The listing builds one solid part. Answer for the finished solid, in the listing's coordinates (mm). Face numbers are marked on the shaded views. Round coordinates to 2 decimals unless told otherwise and drop trailing zeros. Write each loop counter-clockwise with the first axis right and the second up, starting at its lowest first coordinate (ties: lowest second). Pieces come first, ordered by that corner, then holes. Notation, with made-up numbers: (-34.5, -18) - (16.5, -18) arc R19 ccw to (16.5, -10) - close; hole circle Ø9 at (84, -20.5). An arc over 180 degrees is marked (long way). Answer in a Markdown table with one row per item.
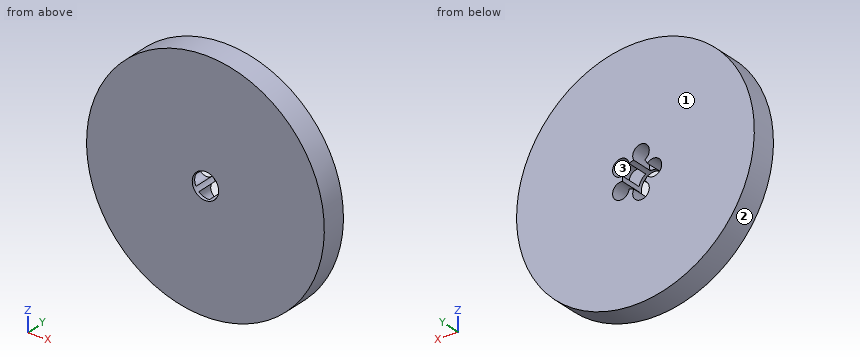
from build123d import *

# Parameters (mm, degrees)
SKETCH1_R           = 90
BOSS_EXTRUDE1_DEPTH = 19
SKETCH2_R           = 10
CUT_EXTRUDE1_DEPTH  = 129.689548915
SKETCH3_R           = 6.277196243
CUT_EXTRUDE2_DEPTH  = 16.549655
CIRPATTERN1_START   = 2.450345027
CIRPATTERN1_DEPTH   = 16.549654973


# Read off the part's stored shape, not the designer's step: CirPattern1
with BuildPart() as part:
    # Sketch1 → Boss-Extrude1 (new body)
    with BuildSketch(Plane(origin=(0, 0, 0), x_dir=(1, 0, 0), z_dir=(0, 1, 0))):
        with Locations(Location((0, 0, 0), (0, 0, 270))):
            Circle(SKETCH1_R)
    extrude(amount=BOSS_EXTRUDE1_DEPTH)

    # Sketch2 → Cut-Extrude1 (cut, through all)
    with BuildSketch(Plane(origin=(0, 0, 0), x_dir=(1, 0, 0), z_dir=(0, 1, 0))):
        with Locations(Location((0, 0, 0), (0, 0, 270))):
            Circle(SKETCH2_R)
    extrude(amount=CUT_EXTRUDE1_DEPTH, mode=Mode.SUBTRACT)

    # Sketch3 → Cut-Extrude2 (cut)
    with BuildSketch(Plane(origin=(0, 19, 0), x_dir=(1, 0, 0), z_dir=(0, 1, 0))):
        with Locations((-13.61267623, 0)):
            Circle(SKETCH3_R)
    extrude(amount=-CUT_EXTRUDE2_DEPTH, mode=Mode.SUBTRACT)

    # CirPattern1 outline → CirPattern1 (cut)
    with BuildSketch(Plane(origin=(0, 0, 0), x_dir=(1, 0, 0), z_dir=(0, 1, 0)).offset(CIRPATTERN1_START)):
        with BuildLine():
            ThreePointArc((1.290880947, -9.916331296), (-3.090169944, -9.510565163), (-6.873017917, -7.263719758))
            ThreePointArc((-6.873017917, -7.263719758), (-6.146308609, -18.916392824), (1.290880947, -9.916331296))
        make_face()
        with BuildLine():
            ThreePointArc((1.290880947, 9.916331296), (-6.146308609, 18.916392824), (-6.873017917, 7.263719758))
            ThreePointArc((-6.873017917, 7.263719758), (-3.090169944, 9.510565163), (1.290880947, 9.916331296))
        make_face()
        with BuildLine():
            ThreePointArc((9.829895648, -1.836614156), (8.090169944, -5.877852523), (4.784328669, -8.781241324))
            ThreePointArc((4.784328669, -8.781241324), (16.091244847, -11.69097371), (9.829895648, -1.836614156))
        make_face()
        with BuildLine():
            ThreePointArc((9.829895648, 1.836614156), (16.091244847, 11.69097371), (4.784328669, 8.781241324))
            ThreePointArc((4.784328669, 8.781241324), (8.090169944, 5.877852523), (9.829895648, 1.836614156))
        make_face()
    extrude(amount=CIRPATTERN1_DEPTH, mode=Mode.SUBTRACT)


solid = part.part
(1) Section B-B (x = 7) is taken. Give the vertices of the cut face in (y, z).
Checked values:
| item | result |
|---|---|
| outline | (0, -89.73) - (19, -89.73) - (19, -12.83) - (2.45, -12.83) - (2.45, -7.14) - (0, -7.14) - close; (0, 7.14) - (2.45, 7.14) - (2.45, 12.83) - (19, 12.83) - (19, 89.73) - (0, 89.73) - close |
(2) Flat-ended cylindrical pins translate along their axes: pin 1 (10 mm diameter, centred on y = 11, z = -34, fed in from -X); pin 2 (6.5 mm diameter, centred on x = 10, z = -8.5, fed in from +Y); pin 3 (8 mm diameter, centred on x = -22, y = 7, fed in from -Z). Find the tip coordinate at first contact, or state that the pin passes through.
Checked values:
| item | result |
|---|---|
| pin 1 | stops at x = -85.2 |
| pin 2 | stops at y = 2.45 |
| pin 3 | stops at z = -88.18 |
(3) Find the intervals of material crossed by line 1 (X direction, y = 12.5, z = 0); line 2 (X direction, y = 16.75, z = 12); line 3 (Z direction, x = 1.5, y = 7.75), in increasing order.
Checked values:
| item | result |
|---|---|
| line 1 | x = -90 to -19.89, 10 to 90 |
| line 2 | x = -89.2 to -10.41, 2 to 6.17, 15.85 to 89.2 |
| line 3 | z = -89.99 to -15.56, -10.33 to -9.89, 9.89 to 10.33, 15.56 to 89.99 |
(4) Section D-D (x = 49) is taken. Give the vertices of the cut face in (y, z).
Checked values:
| item | result |
|---|---|
| outline | (0, -75.49) - (19, -75.49) - (19, 75.49) - (0, 75.49) - close |
(5) Section C-C (z = -74) is taken. Give the vertices of the cut face in (x, y) (3 decimals).
Checked values:
| item | result |
|---|---|
| outline | (-51.225, 0) - (51.225, 0) - (51.225, 19) - (-51.225, 19) - close |
(6) Section A-A (y = 8) is taken. Give the vertices of the cut face in (x, z), and give its area (3 significant figures).
Checked values:
| item | result |
|---|---|
| outline | circle Ø180 at (0, 0); hole (-9.03, -4.29) arc R10 ccw to (-6.87, -7.26) arc R6.28 ccw (long way) to (1.29, -9.92) arc R10 ccw to (4.78, -8.78) arc R6.28 ccw (long way) to (9.83, -1.84) arc R10 ccw to (9.83, 1.84) arc R6.28 ccw (long way) to (4.78, 8.78) arc R10 ccw to (1.29, 9.92) arc R6.28 ccw (long way) to (-6.87, 7.26) arc R10 ccw to (-9.03, 4.29) arc R6.28 ccw (long way) to start |
| area | 24,600 mm2 |
(7) For a pull along Z with two mould halves and no side action, classify the marked faces 1, 2 and 3 as pulls with the +Z half, pulls with the -Z half, needs draft (parallel to the pull), parting line crosses it, or undercut.
Checked values:
| item | result |
|---|---|
| face 1 | needs draft |
| face 2 | parting line crosses it |
| face 3 | undercut |
